Build history of the part. All positions in model axes, mm. A direction names the side the tool comes from. Round coordinates to 2 decimals unless told otherwise and drop trailing zeros. Order: outer loops, then holes, each group sorted by start corner. A loop starts at its lowest first (then second) coordinate and runs counter-clockwise, first axis right, second up. Notation, with made-up numbers: M -37.5,65.25 L -17.5,65.25 A16 cw -17.5,71.25 Z; hole C 80.25,-35.75 d1. An arc over 180 degrees is marked long. One line per item, written item: value. Start each with the question number.
Item 1: Pin check, flat tips, straight feed: pin 1 (8 mm diameter, centred on x = -9, z = -134.5, fed in from -Y); pin 2 (1.5 mm diameter, centred on y = 2, z = -25, fed in from +X); pin 3 (0.9 mm diameter, centred on x = 1, y = 2, fed in from -Z). Stop position of each tip, or through.
Item 2: Tool access for faces 4 (the flat face through (0, 1, -123)), 5 (the flat face through (0, 1, -28)), 6 (the flat face through (-23.5, 1, -45)), 7 (the flat face through (-14, 1, -150)): list every direction of +Z, -Z, +X, -X, +Y, -Y with a clear straight run to the whole face (end or side of a thin tool).
Item 3: Two-plate mould, pull along Z, no slides. Class faces 1 (the flat face through (1, 1, -55)), 2 (the flat face through (2, 1, -95)), 3 (the cylindrical face through (-16.2, 1.52, -91.54)): +Z half, -Z half, draft (parallel to the pull), parting line (faces both ways), or undercut.
Item 4: Probe L1, parallel to Z at x = -18, y = 2.5; L2, parallel to Z at x = -22, y = 2.75; L3, parallel to Z at x = -14.5, y = 2.2. List the from-to ranges inside material, lowest first.
Item 5: Band-saw the part on A-A, the plane x = -18. Write the cut outline in (y, z).
Item 6: Band-saw the part on C-C, the plane z = -12. Write the cut outline in (x, y).
Item 7: Band-saw the part on B-B, the plane y = 2.2. Write the cut outline in (x, z).
Autodesk Inventor part; units mm, degrees
ref_plane "YZ Plane" through (0, 0, 0) normal (1, 0, 0) x (0, 1, 0)
ref_plane "XZ Plane" through (0, 0, 0) normal (0, 1, 0) x (-1, 0, 0)
ref_plane "XY Plane" through (0, 0, 0) normal (0, 0, 1) x (1, 0, 0)
sketch "Sketch1" plane through (0, 0, 0) normal (0, 1, 0) x (-1, 0, 0)
  line L0 (0, 0) -> (28, 0)
  line L1 (28, 0) -> (28, -150)
  line L2 (28, -150) -> (0, -150)
  line L3 (0, -150) -> (0, 0)
  line L4 (0, -55) -> (-3, -55)
  line L5 (-3, -55) -> (-3, -95)
  line L6 (-3, -95) -> (0, -95)
  line L7 (0, -95) -> (0, -55)
  line L8 (28, -75) -> (0, -75) construction
  line L9 (-3, -75) -> (0, -75) construction
  point P0 (0, -95)
  dimension "d0" = 150
  dimension "d1" = 3
  dimension "d2" = 40
  dimension "d3" = 28
extrude "Extrusion1" add sketch "Sketch1" along normal blind 3
sketch "Sketch3" plane through (0, 3, 0) normal (0, 1, 0) x (1, 0, 0)
  circle A0 centre (-18, 95) radius 3.9
  line L0 (-28, 150) -> (-28, 0)
  line L1 (0, 95) -> (0, 150)
  line L2 (-28, 0) -> (0, 0)
  line L3 (0, 150) -> (-28, 150)
  dimension "d18" = 7.8
  dimension "d20" = 18
  dimension "d24" = 55
extrude "Extrusion3" cut sketch "Sketch3" against normal blind 3
sketch "Sketch4" plane through (0, 0, 0) normal (0, -1, 0) x (1, 0, 0)
  line L0 (-10.5, -55) -> (-23.5, -55)
  line L1 (-23.5, -55) -> (-23.5, -35)
  line L2 (-23.5, -35) -> (-10.5, -35)
  line L3 (-10.5, -35) -> (-10.5, -55)
  line L4 (-10.5, -55) -> (-23.5, -35) construction
  line L5 (-23.5, -55) -> (-10.5, -35) construction
  line L6 (-28, 0) -> (0, 0)
  point P0 (-17, -45)
  dimension "d25" = 20
  dimension "d26" = 13
  dimension "d27" = 45
extrude "Extrusion4" cut sketch "Sketch4" against normal blind 10
fillet "Fillet1" radius 2 1 edges at (-28, 1.5, 0)
properties part number "Lateral BNC"
Output:
1. pin 1: stops at y = 0
1. pin 2: stops at x = 0
1. pin 3: stops at z = -95
2. face 4: -Z, +X, +Y, -Y
2. face 5: +Z, +X, +Y, -Y
2. face 6: +Y, -Y
2. face 7: -Z, +X, -X, +Y, -Y
3. face 1: +Z half
3. face 2: -Z half
3. face 3: undercut
4. L1: z = -150 to -98.9, -91.1 to -55, -35 to 0
4. L2: z = -150 to -55, -35 to 0
4. L3: z = -150 to -96.72, -93.28 to -55, -35 to 0
5. outline: M 0,-150 L 3,-150 L 3,-98.9 L 0,-98.9 Z; M 0,-91.1 L 3,-91.1 L 3,-55 L 0,-55 Z; M 0,-35 L 3,-35 L 3,0 L 0,0 Z
6. outline: M -28,0 L 0,0 L 0,3 L -28,3 Z
7. outline: M -28,-150 L 0,-150 L 0,-95 L 3,-95 L 3,-55 L 0,-55 L 0,0 L -26,0 A2 ccw -28,-2 Z; hole M -23.5,-55 L -10.5,-55 L -10.5,-35 L -23.5,-35 Z; hole C -18,-95 d7.8
